```python
from build123d import *

# Parameters (mm, degrees)
SKETCH1_W               = 250
SKETCH1_H               = 250
BOSS_EXTRUDE1_DEPTH     = 28
CUT_EXTRUDE1_REACH      = 180.98
SKETCH2_R               = 105
SKETCH3_W               = 15
SKETCH3_H               = 250
BOSS_EXTRUDE2_DEPTH     = 150
SKETCH4_R               = 40
CUT_EXTRUDE2_DEPTH      = 332.374410599
CUT_EXTRUDE4_DEPTH      = 332.374410599
CUT_EXTRUDE4_DEPTH_BACK = 332.374410599
FILLET1_R               = 5


with BuildPart() as part:
    # Sketch1 → Boss-Extrude1 (new body)
    with BuildSketch(Plane(origin=(0, 0, 0), x_dir=(1, 0, 0), z_dir=(0, 1, 0))):
        Rectangle(SKETCH1_W, SKETCH1_H)
    extrude(amount=BOSS_EXTRUDE1_DEPTH)

    # Sketch2 → Cut-Extrude1 (cut, up to next)
    with BuildSketch(Plane(origin=(0, 28, 0), x_dir=(1, 0, 0), z_dir=(0, 1, 0)), mode=Mode.PRIVATE) as cut_extrude1_sk1:
        with Locations(Location((0, 0, 0), (0, 0, 270))):
            Circle(SKETCH2_R)
    cut_extrude1_tool1 = extrude(cut_extrude1_sk1.sketch, amount=-CUT_EXTRUDE1_REACH, mode=Mode.PRIVATE) & part.part
    add(cut_extrude1_tool1.solids().sort_by_distance((0, 28, 0))[0], mode=Mode.SUBTRACT)

    # Sketch3 → Boss-Extrude2 (add)
    with BuildSketch(Plane(origin=(0, 28, 0), x_dir=(1, 0, 0), z_dir=(0, 1, 0))):
        with Locations((-117.5, 0)):
            Rectangle(SKETCH3_W, SKETCH3_H)
    boss_extrude2 = extrude(amount=BOSS_EXTRUDE2_DEPTH)

    # Mirror1: Boss-Extrude2 across plane
    add(boss_extrude2.mirror(Plane(origin=(0, 0, 0), x_dir=(0, 0, 1), z_dir=(1, 0, 0))))

    # Sketch4 → Cut-Extrude2 (cut, through all)
    with BuildSketch(Plane(origin=(125, 0, 0), x_dir=(0, 0, -1), z_dir=(1, 0, 0))):
        with Locations((0, 104.34)):
            Circle(SKETCH4_R)
    extrude(amount=-CUT_EXTRUDE2_DEPTH, mode=Mode.SUBTRACT)

    # Sketch5 → Cut-Extrude4 (cut, two sides: drawn at the far end of the back side and taken through both)
    with BuildSketch(Plane(origin=(125, 0, 0), x_dir=(0, 0, -1), z_dir=(1, 0, 0)).offset(-CUT_EXTRUDE4_DEPTH_BACK)):
        with BuildLine():
            Line((407.036525122, -493.744479882), (125, 28))
            Line((125, 28), (64.798533304, 139.367784424))
            ThreePointArc((64.798533304, 139.367784424), (0, 178), (-64.798533304, 139.367784424))
            Line((-64.798533304, 139.367784424), (-125, 28))
            Line((-125, 28), (-407.036525122, -493.744479882))
            Line((-407.036525122, -493.744479882), (-407.036525122, 692.445899087))
            Line((-407.036525122, 692.445899087), (407.036525122, 692.445899087))
            Line((407.036525122, 692.445899087), (407.036525122, -493.744479882))
        make_face()
    extrude(amount=CUT_EXTRUDE4_DEPTH + CUT_EXTRUDE4_DEPTH_BACK, mode=Mode.SUBTRACT)

    # Fillet1
    fillet1_edges = [part.edges().sort_by_distance(p)[0] for p in [
        (125, 14, 125),
        (-125, 14, 125),
        (-125, 14, -125),
        (125, 14, -125),
    ]]
    fillet(fillet1_edges, radius=FILLET1_R)


solid = part.part
```
Geometry check sheet. Reference: the model listing, model coordinates, mm. A direction names the side the tool comes from. Round coordinates to 2 decimals unless told otherwise and drop trailing zeros. Order: outer loops, then holes, each group sorted by start corner. A loop starts at its lowest first (then second) coordinate and runs counter-clockwise, first axis right, second up. Notation, with made-up numbers: (-35, -7) -> (18, -7) arc R16 cw to (18, 0) -> close; hole circle Ø11 at (13, 16). An arc over 180 degrees is marked (long way). Return JSON: item names as keys, results as strings. Group by question number.
Q1. Tool access check on faces 5 (the flat face through (-117.605, 82.904, -95.321)), 6 (the flat face through (-110, 69, -26)). Record the directions out of +Z, -Z, +X, -X, +Y, -Y that give a thin tool (end or side, any length) a straight path to the whole face; none if there is none.
Q2. Section check D-D, the plane z = -77. Record the boundary of the cut face in (x, y), plus the area to 3 significant figures.
Q3. Section check A-A, the plane x = 0. Record the boundary of the cut face in (y, z).
Q4. Release check for a two-part mould opening along X. For faces 1 (the flat face through (110, 69, -26)), 2 (the flat face through (125, 48, 2)), 3 (the flat face through (-75, 28, -85)), 4 (the flat face through (-113, 0, -2)) record: released by +X, released by -X, zero draft, split by the parting line, or undercut.
Q5. Gauge pin test, flat end, axial feed: pin 1 (12 mm diameter, centred on x = 61.5, z = 93.5, fed in from +Y). Record the tip position at first contact, or that the pin passes through.
Q6. Material ranges on probe 1 along Y at (x, z) = (-114, 0); probe 2 along X at (y, z) = (12, 0); probe 3 along X at (y, z) = (43.5, -78), recorded low to high. Write a range as from..to.
Q7. Section check B-B, the plane z = 0. Record the boundary of the cut face in (x, y).
Q8. Section check C-C, the plane y = 126. Record the boundary of the cut face in (x, z), plus the area to 3 significant figures.
Numbers:
{
 "1": {"face 5": "-Z, +X, -X, +Y", "face 6": "+Z, -Z, +Y"},
 "2": {"outline": "(-125, 0) -> (-71.39, 0) -> (-71.39, 28) -> (-110, 28) -> (-110, 116.8) -> (-125, 116.8) -> close; (71.39, 0) -> (125, 0) -> (125, 116.8) -> (110, 116.8) -> (110, 28) -> (71.39, 28) -> close", "area": "5,670 mm^2"},
 "3": {"outline": "(0, -125) -> (28, -125) -> (28, -105) -> (0, -105) -> close; (0, 105) -> (28, 105) -> (28, 125) -> (0, 125) -> close"},
 "4": {"face 1": "undercut", "face 2": "released by +X", "face 3": "undercut", "face 4": "zero draft"},
 "5": {"pin 1": "y = 28"},
 "6": {"probe 1": "0..64.34, 144.34..178", "probe 2": "-125..-105, 105..125", "probe 3": "-125..-110, 110..125"},
 "7": {"outline": "(-125, 0) -> (-105, 0) -> (-105, 28) -> (-110, 28) -> (-110, 64.34) -> (-125, 64.34) -> close; (-125, 144.34) -> (-110, 144.34) -> (-110, 178) -> (-125, 178) -> close; (105, 0) -> (125, 0) -> (125, 64.34) -> (110, 64.34) -> (110, 28) -> (105, 28) -> close; (110, 144.34) -> (125, 144.34) -> (125, 178) -> (110, 178) -> close"},
 "8": {"outline": "(-125, -72.02) -> (-110, -72.02) -> (-110, -33.63) -> (-125, -33.63) -> close; (-125, 33.63) -> (-110, 33.63) -> (-110, 72.02) -> (-125, 72.02) -> close; (110, -72.02) -> (125, -72.02) -> (125, -33.63) -> (110, -33.63) -> close; (110, 33.63) -> (125, 33.63) -> (125, 72.02) -> (110, 72.02) -> close", "area": "2,300 mm^2"}
}
